Can you work these out from the model? Positions are in its coordinate system, mm. Face numbers are marked on the shaded views. A direction names the side the tool comes from. Round coordinates to 2 decimals unless told otherwise and drop trailing zeros. Loops run counter-clockwise (first coordinate to the right, second up) from the corner with the lowest first, then second, coordinate; pieces in that order, holes last. Notation, with made-up numbers: (17.5, -17.5) -> (43.5, -17.5) arc R13 ccw to (43.5, -9.5) -> close; hole circle Ø2 at (80, -9.5). An arc over 180 degrees is marked (long way). Write item = value, one per line.
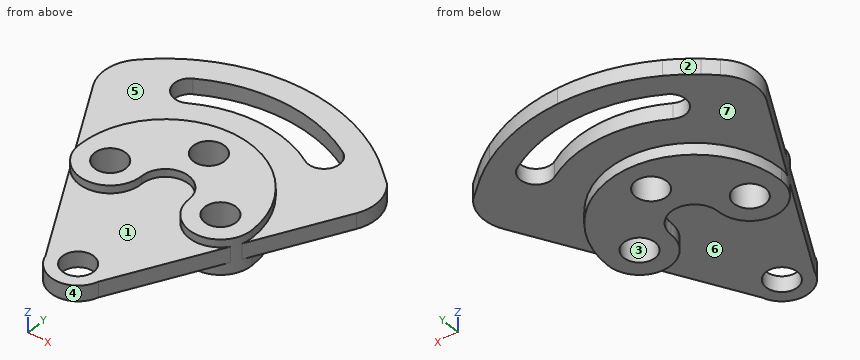
Autodesk Inventor part; units mm, degrees
ref_plane "YZ Plane" through (0, 0, 0) normal (1, 0, 0) x (0, 1, 0)
ref_plane "XZ Plane" through (0, 0, 0) normal (0, 1, 0) x (-1, 0, 0)
ref_plane "XY Plane" through (0, 0, 0) normal (0, 0, 1) x (1, 0, 0)
sketch "Эскиз1" plane through (0, 0, 0) normal (0, 0, 1) x (1, 0, 0)
  circle A0 centre (0, 0) radius 17.5
  circle A1 centre (0, 0) radius 10
  line L0 (0, 0) -> (0, 70)
  arc A2 (35, 70) -> (-35, 70) centre (0, 70) ccw
  arc A3 (55, 70) -> (-55, 70) centre (0, 70) ccw
  arc A4 (15, 70) -> (-15, 70) centre (0, 70) ccw
  arc A5 (-55, 70) -> (-15, 70) centre (-35, 70) ccw
  arc A6 (15, 70) -> (55, 70) centre (35, 70) ccw
  circle A7 centre (-35, 70) radius 10
  circle A8 centre (0, 105) radius 10
  circle A9 centre (35, 70) radius 10
  line L1 (-35, 70) -> (-35, 50)
  line L2 (-35, 50) -> (-35, 44.4464)
  line L3 (35, 70) -> (35, 50)
  line L4 (35, 50) -> (35, 44.4464)
  arc A10 (55, 165.2628) -> (0, 180) centre (0, 70) ccw
  line L5 (0, 70) -> (55, 165.2628) construction
  line L6 (0, 70) -> (0, 180) construction
  arc A11 (0, 180) -> (-55, 165.2628) centre (0, 70) ccw
  line L7 (0, 70) -> (-55, 165.2628) construction
  line L8 (0, 70) -> (0, 180) construction
  arc A12 (42.5, 143.6122) -> (-42.5, 143.6122) centre (0, 70) ccw
  arc A13 (37.5, 134.9519) -> (47.5, 152.2724) centre (42.5, 143.6122) ccw
  arc A14 (-47.5, 152.2724) -> (-37.5, 134.9519) centre (-42.5, 143.6122) ccw
  arc A15 (47.5, 152.2724) -> (-47.5, 152.2724) centre (0, 70) ccw
  arc A16 (37.5, 134.9519) -> (-37.5, 134.9519) centre (0, 70) ccw
  line L9 (0, 0) -> (-17.5, 0)
  line L10 (0, 0) -> (17.5, 0)
  line L11 (0, 0) -> (-10, 0)
  line L12 (0, 0) -> (10, 0)
  line L13 (0, 70) -> (0, 180)
  arc A17 (-55, 165.2628) -> (-70.7066, 154.2649) centre (0, 70) ccw
  line L14 (0, 70) -> (-55, 165.2628) construction
  line L15 (0, 70) -> (55, 165.2628)
  arc A18 (70.764, 154.2167) -> (55, 165.2628) centre (0, 70) ccw
  line L16 (-16.7681, -5.0081) -> (-83.5023, 117.8971)
  arc A19 (-70.7066, 154.2649) -> (-77.7825, 147.781) centre (0, 70) ccw
  arc A20 (-77.7825, 147.781) -> (-83.5023, 117.8971) centre (-61.1578, 129.1097) ccw
  line L17 (16.7749, -4.9852) -> (83.4973, 117.9265)
  line L18 (70.764, 154.2167) -> (80.7777, 145.8026)
  arc A21 (83.4973, 117.9265) -> (80.7777, 145.8026) centre (61.5259, 129.8537) ccw
  dimension "d15" = 70
  dimension "d17" = 105
  dimension "d19" = 30
  dimension "d20" = 30
  dimension "d23" = 10
  dimension "d28" = 35
  dimension "d29" = 20
  dimension "d30" = 20
  dimension "d31" = 15
  dimension "d32" = 35
  dimension "d33" = 85
  dimension "d34" = 110
  dimension "d35" = 55
  dimension "d55" = 25
  dimension "d110" = 19.5925
  dimension "d111" = 107.0482
  dimension "d112" = 152.0798
  dimension "d113" = 104.0886
  dimension "d114" = 90.9725
  dimension "d115" = 101.544
  dimension "d116" = 49.961
  dimension "d117" = 21.46
  dimension "d119" = 17.1211
  dimension "d120" = 17.1257
extrude "Выдавливание1" add sketch "Эскиз1" along normal blind 10 contours L9 A1 L10 A0 | A0 L16 A5 A4 L13 L0 | A0 L0 A1 L9 | L0 L15 A4 A6 L17 A0 | A0 L10 A1 L0 | L16 A5 A3 L13 A8 A2 A7 L1 | L13 A4 L15 | A6 L3 A9 A2 L15 A3 L17 | L16 A20 A19 A17 A11 L13 A15 A14 A16 A3 A5 | L1 A7 A2 A8 L13 A4 A5 | L13 A8 A2 L15 A4 | L15 A2 A9 L3 A6 A4 | A6 A3 L15 A13 A18 L18 A21 L17 | A2 A8 L13 A3 L15 | L13 A16 L15 A3 | A15 L13 A10 L15
extrude "Выдавливание2" add sketch "Эскиз1" along normal blind 15 and the other way blind 7.5 contours L16 A5 A3 L13 A8 A2 A7 L1 | A5 L16 | L17 A6 | A6 L3 A9 A2 L15 A3 L17 | L1 A7 A2 A8 L13 A4 A5 | L13 A8 A2 L15 A4 | L15 A2 A9 L3 A6 A4 | A2 A8 L13 A3 L15
properties part number "lab2_1_2"
1. Suppose I cut it at C-C, the plane x = 5.5. List the corners of the cut face in (y, z) for me, and give its area (3 significant figures).
Entries:
outline = (-16.61, 0) -> (-8.35, 0) -> (-8.35, 10) -> (-16.61, 10) -> close; (8.35, 0) -> (83.96, 0) -> (83.96, -7.5) -> (96.65, -7.5) -> (96.65, 15) -> (83.96, 15) -> (83.96, 10) -> (8.35, 10) -> close; (113.35, -7.5) -> (124.72, -7.5) -> (124.72, 0) -> (144.8, 0) -> (144.8, 10) -> (124.72, 10) -> (124.72, 15) -> (113.35, 15) -> close; (164.84, 0) -> (179.86, 0) -> (179.86, 10) -> (164.84, 10) -> close
area = 1,730 mm²
2. I'm going to push flat-ended pins straight in: pin 1 (4 mm diameter, centred on y = 26, z = 3.5, fed in from -X); pin 2 (1 mm diameter, centred on y = 6, z = 7, fed in from -X); pin 3 (4 mm diameter, centred on x = 17.5, z = 7, fed in from -Y); pin 4 (23 mm diameter, centred on x = 0, y = 105, fed in from -Z). Where does each tip first touch, or does it pass through?
Entries:
pin_1 = -34.69
pin_2 = -23.02
pin_3 = -8.12
pin_4 = -7.5
3. We'd pull the mould along Y, two halves only. Please class the marked faces 1, 2, 3 and 4: released by +Y, released by -Y, zero draft, split by the parting line, or undercut.
Entries:
face_1 = zero draft
face_2 = released by +Y
face_3 = undercut
face_4 = released by -Y
4. Suppose I cut it at A-A, the plane z = -3. List the corners of the cut face in (x, y) for me, and give its area (3 significant figures).
Entries:
outline = (-55, 70) arc R20 ccw to (-15, 70) arc R15 cw to (15, 70) arc R20 ccw to (55, 70) arc R55 ccw to start; hole circle Ø20 at (-35, 70); hole circle Ø20 at (0, 105); hole circle Ø20 at (35, 70)
area = 4,710 mm²
5. Suppose I cut it at B-B, the plane y = 105. List the corners of the cut face in (x, z) for me, and give its area (3 significant figures).
Entries:
outline = (-76.5, 0) -> (-42.43, 0) -> (-42.43, -7.5) -> (-10, -7.5) -> (-10, 15) -> (-42.43, 15) -> (-42.43, 10) -> (-76.5, 10) -> close; (10, -7.5) -> (42.43, -7.5) -> (42.43, 0) -> (76.48, 0) -> (76.48, 10) -> (42.43, 10) -> (42.43, 15) -> (10, 15) -> close
area = 2,140 mm²
6. Suppose I cut it at D-D, the plane y = 141.5. List the corners of the cut face in (x, z) for me.
Entries:
outline = (-82.87, 0) -> (-52.27, 0) -> (-52.27, 10) -> (-82.87, 10) -> close; (-22.64, 0) -> (22.64, 0) -> (22.64, 10) -> (-22.64, 10) -> close; (52.27, 0) -> (83.65, 0) -> (83.65, 10) -> (52.27, 10) -> close
7. I need wall thicknesses on line 1 (Y direction, x = 0, z = 7.5); line 2 (Y direction, x = 35, z = 0.25); line 3 (Y direction, x = -43, z = 7.5). Which ranges of each line are inside material? Lowest first, please. Write a range as [from, to].
Entries:
line_1 = [-17.5, -10], [10, 95], [115, 145], [165, 180]
line_2 = [28.59, 60], [80, 136.33], [158.32, 174.28]
line_3 = [43.3, 64], [76, 133.62], [154.71, 171.25]
8. For the marked faces 5, 6 and 7, which set-ups out of +Z, -Z, +X, -X, +Y, -Y let a thin tool reach every point of the face, with its end or its side?
Entries:
face_5 = +Z, +Y
face_6 = -Z, -Y
face_7 = -Z, +Y
